Can you work these out from the model? Positions are in its coordinate system, mm. Face numbers are marked on the shaded views. A direction names the side the tool comes from. Give positions to 0.01 mm unless a question says otherwise; leave off trailing zeros. Loops run counter-clockwise (first coordinate to the right, second up) from the corner with the lowest first, then second, coordinate; pieces in that order, holes last. Notation, with made-up numbers: M -23.5,27.5 L 22.5,27.5 A19 cw 22.5,35.5 Z; hole C 45,-4 d6. An arc over 180 degrees is marked long. Answer as a JSON object with one key per item and string values.
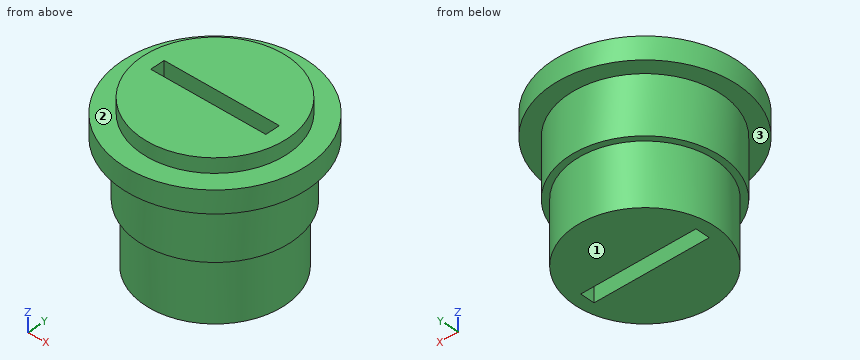
```python
from build123d import *

# Parameters (mm, degrees)
F2_R     = 17
F3_DEPTH = 15
F4_W     = 28
F4_H     = 3.5
F5_DEPTH = 40


with BuildPart() as f1:
    # F0 (on Front) → F1 (revolve)
    with BuildSketch(Plane.XZ):
        Polygon((0, 22.9), (0, 0), (18.5, 0), (18.5, 14), (22.5, 14), (22.5, 19.4), (17.64, 19.4), (17.64, 22.9), align=None)
    revolve(axis=Axis((0, 0, -1.557709), (0, 0, 1)))

    # F2 (on face) → F3 (join)
    with BuildSketch(Plane(origin=(0, 0, 0), x_dir=(1, 0, 0), z_dir=(0, 0, -1))):
        Circle(F2_R)
    extrude(amount=F3_DEPTH)

    # F4 (on face) → F5 (cut)
    with BuildSketch(Plane(origin=(0, 0, -15), x_dir=(1, 0, 0), z_dir=(0, 0, -1))):
        Rectangle(F4_W, F4_H)
    extrude(amount=-F5_DEPTH, mode=Mode.SUBTRACT)


solid = f1.part
```
1) Suppose I cut it at C-C, the plane z = 1. Write out the boundary of the cut face in (x, y).
Answer list:
{"outline": "C 0,0 d37; hole M -14,-1.75 L 14,-1.75 L 14,1.75 L -14,1.75 Z"}
2) For the marked faces 1, 2 and 3, which set-ups out of +Z, -Z, +X, -X, +Y, -Y let a thin tool reach every point of the face, with its end or its side?
Answer list:
{"face 1": "-Z, +X, -X, +Y, -Y", "face 2": "+Z", "face 3": "-Z"}
3) Please list where these lines run through material, in increasing order: line 1 along Z through (x, y) = (20, 8.5); line 2 along Y through (x, z) = (-8.5, -4); line 3 along Y through (x, z) = (2, -11.5). Write a range as from..to.
Answer list:
{"line 1": "14..19.4", "line 2": "-14.72..-1.75, 1.75..14.72", "line 3": "-16.88..-1.75, 1.75..16.88"}
4) Suppose I cut it at D-D, the plane y = -14. Write out the boundary of the cut face in (x, z), and give its area (3 significant figures).
Answer list:
{"outline": "M -17.61,14 L -12.09,14 L -12.09,0 L -9.64,0 L -9.64,-15 L 9.64,-15 L 9.64,0 L 12.09,0 L 12.09,14 L 17.61,14 L 17.61,19.4 L 10.73,19.4 L 10.73,22.9 L -10.73,22.9 L -10.73,19.4 L -17.61,19.4 Z", "area": "893 mm^2"}
5) Will these pins go through, and if not, where does the flat tip stop? pin 1 Ø22.5 at (x, z) = (3, 8.5) entering from -Y; pin 2 Ø8.5 at (x, z) = (6.5, 6.5) entering from +Y; pin 3 Ø8 at (x, z) = (8, 1) entering from +Y.
Answer list:
{"pin 1": "y = -22.5", "pin 2": "y = 18.36", "pin 3": "y = 18.06"}
6) Suppose I cut it at B-B, the plane y = 0. Write out the boundary of the cut face in (x, z), and give its area (3 significant figures).
Answer list:
{"outline": "M -22.5,14 L -18.5,14 L -18.5,0 L -17,0 L -17,-15 L -14,-15 L -14,22.9 L -17.64,22.9 L -17.64,19.4 L -22.5,19.4 Z; M 14,-15 L 17,-15 L 17,0 L 18.5,0 L 18.5,14 L 22.5,14 L 22.5,19.4 L 17.64,19.4 L 17.64,22.9 L 14,22.9 Z", "area": "333 mm^2"}
7) Suppose I cut it at A-A, the plane x = 0. Write out the boundary of the cut face in (y, z), and give its area (3 significant figures).
Answer list:
{"outline": "M -22.5,14 L -18.5,14 L -18.5,0 L -17,0 L -17,-15 L -1.75,-15 L -1.75,22.9 L -17.64,22.9 L -17.64,19.4 L -22.5,19.4 Z; M 1.75,-15 L 17,-15 L 17,0 L 18.5,0 L 18.5,14 L 22.5,14 L 22.5,19.4 L 17.64,19.4 L 17.64,22.9 L 1.75,22.9 Z", "area": "1,260 mm^2"}
